```python
from build123d import *

# Parameters (mm, degrees)
BOSS_EXTRUDE1_DEPTH = 2
SKETCH2_R           = 2
BOSS_EXTRUDE2_DEPTH = 8
SKETCH5_R           = 2
CUT_EXTRUDE2_DEPTH  = 4
BOSS_EXTRUDE3_DEPTH = 2
CUT_EXTRUDE1_DEPTH  = 5.5


with BuildPart() as part:
    # Sketch1 → Boss-Extrude1 (new body)
    with BuildSketch(Plane.XY):
        with BuildLine():
            Line((0, -2.5), (34, -2.5))
            ThreePointArc((34, -2.5), (36.5, 0), (34, 2.5))
            Line((34, 2.5), (0, 2.5))
            ThreePointArc((0, 2.5), (-2.5, 0), (0, -2.5))
        make_face()
    extrude(amount=BOSS_EXTRUDE1_DEPTH)

    # Sketch2 → Boss-Extrude2 (add)
    with BuildSketch(Plane.XY.offset(2)):
        Circle(SKETCH2_R)
    extrude(amount=BOSS_EXTRUDE2_DEPTH)

    # Sketch5 → Cut-Extrude2 (cut, symmetric)
    with BuildSketch(Plane(origin=(0, 0, 0), x_dir=(-1, 0, 0), z_dir=(0, 0, -1))):
        with Locations(Location((-34, 0, 0), (0, 0, 180))):
            Circle(SKETCH5_R)
    extrude(amount=CUT_EXTRUDE2_DEPTH, both=True, mode=Mode.SUBTRACT)

    # Sketch3 → Boss-Extrude3 (add)
    with BuildSketch(Plane(origin=(0, 0, 0), x_dir=(-1, 0, 0), z_dir=(0, 0, -1))):
        with BuildLine():
            Line((-34, -4.5), (-31.853983948, -4.5))
            ThreePointArc((-31.853983948, -4.5), (-29.476132044, -4.213177664), (-27.234684348, -3.369164065))
            Line((-27.234684348, -3.369164065), (-26.000115193, -2.726167187))
            ThreePointArc((-26.000115193, -2.726167187), (-25.551825654, -2.557364467), (-25.076255273, -2.5))
            Line((-25.076255273, -2.5), (-25.076255273, 2.5))
            ThreePointArc((-25.076255273, 2.5), (-25.551825654, 2.557364467), (-26.000115193, 2.726167187))
            Line((-26.000115193, 2.726167187), (-27.234684348, 3.369164065))
            ThreePointArc((-27.234684348, 3.369164065), (-29.476132044, 4.213177664), (-31.853983948, 4.5))
            Line((-31.853983948, 4.5), (-34, 4.5))
            ThreePointArc((-34, 4.5), (-38.5, 0), (-34, -4.5))
        make_face()
    boss_extrude3 = extrude(amount=BOSS_EXTRUDE3_DEPTH)

    # Sketch4 → Cut-Extrude1 (cut, symmetric)
    with BuildSketch(Plane(origin=(0, 0, 0), x_dir=(1, 0, 0), z_dir=(0, 1, 0))):
        with BuildLine():
            Line((31.853983948, 2), (31.853983948, 3.174344261))
            Line((31.853983948, 3.174344261), (24.383890118, 3.174344261))
            Line((24.383890118, 3.174344261), (25.076255273, 0))
            add(Edge.make_bspline(
                [(31.853983948, 2), (29.962456018, 2.02071595), (29.16990367, 1.605069608), (25.966821868, 0.283607958), (25.076255273, 0)],
                knots=[0, 0, 0, 0, 0.608348739, 1, 1, 1, 1], degree=3))
        make_face()
    cut_extrude1 = extrude(amount=CUT_EXTRUDE1_DEPTH, both=True, mode=Mode.SUBTRACT)

    # Mirror1: Boss-Extrude3, Cut-Extrude1 across plane
    add(boss_extrude3.mirror(Plane.XY.offset(1)))
    add(cut_extrude1.mirror(Plane.XY.offset(1)), mode=Mode.SUBTRACT)


solid = part.part
```
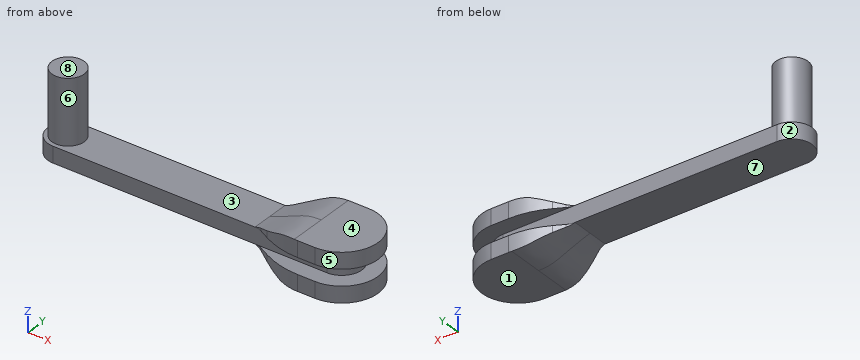
Geometry check sheet. Reference: the model listing, model coordinates, mm. Face numbers are marked on the shaded views. A direction names the side the tool comes from. Coordinates: 2 decimals unless noted, no trailing zeros. Write each loop counter-clockwise with the first axis right and the second up, starting at its lowest first coordinate (ties: lowest second). Pieces come first, ordered by that corner, then holes. Notation, with made-up numbers: M -37,-38.75 L -6,-38.75 A14 cw -6,-18.75 Z; hole C 69,59.25 d9. An arc over 180 degrees is marked long. Answer as a JSON object with one key per item and string values.
1. Draft check along X on the marked faces 1, 2 and 3. Enter one of: released by +X, released by -X, zero draft, split by the parting line, or undercut.
Answers below:
{"face 1": "zero draft", "face 2": "released by -X", "face 3": "undercut"}
2. Section check B-B, the plane z = 8.5. Enter the section's corners in (x, y).
Answers below:
{"outline": "C 0,0 d4"}
3. Tool access check on the marked faces 4, 5, 6, 7 and 8. Record the directions out of +Z, -Z, +X, -X, +Y, -Y that give a thin tool (end or side, any length) a straight path to the whole face; none if there is none.
Answers below:
{"face 4": "+Z, +X, +Y, -Y", "face 5": "+Z, -Z, +X", "face 6": "+Z", "face 7": "-Z, -X, +Y, -Y", "face 8": "+Z, +X, -X, +Y, -Y"}
4. Section check C-C, the plane x = 12. Enter the section's corners in (y, z), plus the area to 3 significant figures.
Answers below:
{"outline": "M -2.5,0 L 2.5,0 L 2.5,2 L -2.5,2 Z", "area": "10.0 mm²"}
5. Scan lines: L1, parallel to Y at x = 34, z = 1.15; L2, parallel to Z at x = 34, y = 1; L3, parallel to Z at x = 9.5, y = 0. Record each from-to range of solid material in increasing order.
Answers below:
{"L1": "y = -2.5 to -2, 2 to 2.5", "L2": "z = -2 to 0, 2 to 4", "L3": "z = 0 to 2"}
6. Go/stop test with flat-tipped pins: pin 1 Ø4 at (x, y) = (9.5, -2) entering from +Z; pin 2 Ø1.5 at (x, z) = (16, 4.5) entering from -Y; pin 3 Ø1 at (x, z) = (1.5, 7) entering from -Y; pin 4 Ø1.6 at (x, z) = (22, 1.5) entering from -Y. Record where each tip stops, or that it passes through.
Answers below:
{"pin 1": "stops at z = 2", "pin 2": "passes through", "pin 3": "stops at y = -1.73", "pin 4": "stops at y = -2.5"}
7. Section check A-A, the plane z = 1. Enter the section's corners in (x, y).
Answers below:
{"outline": "M 0,-2.5 L 34,-2.5 A2.5 ccw 34,2.5 L 0,2.5 A2.5 ccw Z; hole C 34,0 d4"}
